```python
from build123d import *

# Parameters (mm, degrees)
F1_DEPTH = 6.35
F0_R     = 16.612306
F2_DEPTH = 19.05
F3_DEPTH = 31.75
F4_R     = 4.66369
F5_DEPTH = 13.156878


with BuildPart() as f1:
    # F0 (on Front) → F1 (new body)
    with BuildSketch(Plane.XZ):
        with BuildLine():
            Line((22.07386, -42.633548), (22.07386, 0))
            ThreePointArc((22.07386, 0), (0, -22.07386), (-22.07386, 0))
            Line((-22.07386, 0), (-22.07386, -42.633548))
            ThreePointArc((-22.07386, -42.633548), (-33.852086, -72.074216), (-62.68657, -85.267097))
            Line((-62.68657, -85.267097), (-22.07386, -85.267097))
            Line((-22.07386, -85.267097), (22.07386, -85.267097))
            Line((22.07386, -85.267097), (62.68657, -85.267097))
            ThreePointArc((62.68657, -85.267097), (33.852086, -72.074216), (22.07386, -42.633548))
        make_face()
    extrude(amount=F1_DEPTH)

    # F0 (on Front) → F2 (join)
    with BuildSketch(Plane.XZ):
        with BuildLine():
            ThreePointArc((-22.07386, 0), (0, -22.07386), (22.07386, 0))
            ThreePointArc((22.07386, 0), (0, 22.07386), (-22.07386, 0))
        make_face()
        Circle(F0_R, mode=Mode.SUBTRACT)
    extrude(amount=F2_DEPTH)

    # F0 (on Front) → F3 (join)
    with BuildSketch(Plane.XZ):
        Polygon((62.68657, -98.422974), (62.68657, -85.267097), (22.07386, -85.267097), (-22.07386, -85.267097), (-62.68657, -85.267097), (-62.68657, -98.422974), align=None)
    extrude(amount=F3_DEPTH)

    # F4 (on face) → F5 (cut, through all)
    with BuildSketch(Plane.XY.offset(-85.267097)):
        with Locations((-49.98657, -19.05)):
            Circle(F4_R)
        with Locations((49.98657, -19.05)):
            Circle(F4_R)
        with BuildLine():
            Line((-62.68657, -19.05), (-62.68657, -31.75))
            Line((-62.68657, -31.75), (-49.98657, -31.75))
            ThreePointArc((-49.98657, -31.75), (-58.966826, -28.030256), (-62.68657, -19.05))
        make_face()
        with BuildLine():
            ThreePointArc((62.68657, -19.05), (58.966826, -28.030256), (49.98657, -31.75))
            Line((49.98657, -31.75), (62.68657, -31.75))
            Line((62.68657, -31.75), (62.68657, -19.05))
        make_face()
    extrude(amount=-F5_DEPTH, mode=Mode.SUBTRACT)


solid = f1.part
```
Can you work these out from the model? Positions are in its coordinate system, mm. A direction names the side the tool comes from. Coordinates: 2 decimals unless noted, no trailing zeros. Loops run counter-clockwise (first coordinate to the right, second up) from the corner with the lowest first, then second, coordinate; pieces in that order, holes last.
1) Imagine slicing it at D-D on z = -4. List the corners of the cut face in (x, y) for me.
2) Imagine slicing it at A-A on x = 0. List the corners of the cut face in (y, z) for me, plus the area to 3 significant figures.
3) For pin 1 (5 mm diameter, centred on x = -13.5, y = -21, fed in from +Z); pin 2 (22 mm diameter, centred on x = 7, z = 5.5, fed in from -Y); pin 3 (1.9 mm diameter, centred on y = -2.5, z = -11.5, fed in from -X); pin 4 (8 mm diameter, centred on x = 46.5, y = -16, fed in from -Z), each with a flat end and sliding along its axis, tell me the tip position at first contact or that it passes through.
4) Imagine slicing it at C-C on y = -8.5. List the corners of the cut face in (x, z) for me.
5) I need wall thicknesses on probe 1 along X at (y, z) = (-19, -95); probe 2 along Z at (x, y) = (-6, -14); probe 3 along Z at (x, y) = (-2.5, -11). Which ranges of each line are inside material? Lowest first, please.
6) Which directions (+Z, -Z, +X, -X, +Y, -Y) give clear straight access to the entire face, cutting with the end or side of a thin tool? Please do faces 4 (the flat face through (-22.074, -3, -21)), 5 (the cylindrical face through (-2.874, -11.508, 21.886)), 6 (the flat face through (3.2, -19.05, 16.5)).
7) Thinking about a two-plate mould opening in Z: for faces 1 (the flat face through (1, -19, -85.267)), 2 (the flat face through (-1, -16, -98.423)), 3 (the flat face through (62.687, -9, -92)), which applies, pulls with the +Z half, pulls with the -Z half, needs draft (parallel to the pull), parting line crosses it, or undercut?
8) Imagine slicing it at B-B on y = -1.5. List the corners of the cut face in (x, z) for me.
Completed:
1. outline: (-22.07, -6.35) - (-21.71, -6.35) - (-21.71, -19.05) - (-16.12, -19.05) - (-16.12, 0) - (-22.07, 0) - close; (16.12, -19.05) - (21.71, -19.05) - (21.71, -6.35) - (22.07, -6.35) - (22.07, 0) - (16.12, 0) - close
2. outline: (-31.75, -98.42) - (0, -98.42) - (0, -16.61) - (-19.05, -16.61) - (-19.05, -22.07) - (-6.35, -22.07) - (-6.35, -85.27) - (-31.75, -85.27) - close; (-19.05, 16.61) - (0, 16.61) - (0, 22.07) - (-19.05, 22.07) - close
2. area: 1,030 mm2
3. pin 1: stops at z = 18.57
3. pin 2: stops at y = -19.05
3. pin 3: stops at x = -22.07
3. pin 4: stops at z = -98.42
4. outline: (-62.69, -98.42) - (62.69, -98.42) - (62.69, -85.27) - (-62.69, -85.27) - close; circle Ø44.15 at (0, 0); hole circle Ø33.22 at (0, 0)
5. probe 1: x = -62.69 to -54.65, -45.32 to 45.32, 54.65 to 62.69
5. probe 2: z = -98.42 to -85.27, -21.24 to -15.49, 15.49 to 21.24
5. probe 3: z = -98.42 to -85.27, -21.93 to -16.42, 16.42 to 21.93
6. face 4: +Z, -X, +Y, -Y
6. face 5: -Y
6. face 6: +Z, +X, -X, -Y
7. face 1: undercut
7. face 2: pulls with the -Z half
7. face 3: needs draft
8. outline: (-62.69, -98.42) - (62.69, -98.42) - (62.69, -85.27) arc R42.68 cw to (22.07, -42.63) - (22.07, 0) arc R22.07 ccw to (-22.07, 0) - (-22.07, -42.63) arc R42.68 cw to (-62.69, -85.27) - close; hole circle Ø33.22 at (0, 0)
